Geometry check sheet. Reference: the model listing, model coordinates, mm. A direction names the side the tool comes from. Round coordinates to 2 decimals unless told otherwise and drop trailing zeros. Write each loop counter-clockwise with the first axis right and the second up, starting at its lowest first coordinate (ties: lowest second). Pieces come first, ordered by that corner, then holes. Notation, with made-up numbers: (20, 28.5) -> (37, 28.5) arc R14 cw to (37, 43.5) -> close; hole circle Ø3 at (4, 13). An arc over 180 degrees is marked (long way). Use a Markdown table: item, result.
```python
from build123d import *

# Parameters (mm, degrees)
BOSS_EXTRUDE1_DEPTH = 36
SKETCH2_R           = 1.6
CUT_EXTRUDE1_DEPTH  = 10
SKETCH3_R           = 1.95
CUT_EXTRUDE2_DEPTH  = 3
FILLET1_R           = 1
SKETCH4_W           = 8
SKETCH4_H           = 10.3
CUT_EXTRUDE3_DEPTH  = 10
SKETCH5_W           = 5.039372534
SKETCH5_H           = 10.3
CUT_EXTRUDE4_DEPTH  = 10


with BuildPart() as part:
    # Sketch1 → Boss-Extrude1 (new body)
    with BuildSketch(Plane.XY):
        Polygon((1.933806537, 5.15), (1.933806537, -5.15), (0.476512405, -5.15), (-2.040358106, -2.633129489), (-2.040358106, 2.633129489), (0.476512405, 5.15), align=None)
    extrude(amount=BOSS_EXTRUDE1_DEPTH)

    # Sketch2 → Cut-Extrude1 (cut)
    with BuildSketch(Plane(origin=(1.933806537, 0, 0), x_dir=(0, 0, -1), z_dir=(1, 0, 0))):
        with Locations((-16, 0)):
            Circle(SKETCH2_R)
        with Locations((-31, 0)):
            Circle(SKETCH2_R)
        with Locations((-6, 0)):
            Circle(SKETCH2_R)
    extrude(amount=-CUT_EXTRUDE1_DEPTH, mode=Mode.SUBTRACT)

    # Sketch3 → Cut-Extrude2 (cut)
    with BuildSketch(Plane.ZY.offset(2.040358106)):
        with Locations((16, 0)):
            Circle(SKETCH3_R)
        with Locations((31, 0)):
            Circle(SKETCH3_R)
        with Locations((6, 0)):
            Circle(SKETCH3_R)
    extrude(amount=-CUT_EXTRUDE2_DEPTH, mode=Mode.SUBTRACT)

    # Fillet1
    fillet1_edges = [part.edges().sort_by_distance(p)[0] for p in [
        (0.476512405, 5.15, 18),
        (0.476512405, -5.15, 18),
        (-2.040358106, 2.633129489, 18),
        (-2.040358106, -2.633129489, 18),
    ]]
    fillet(fillet1_edges, radius=FILLET1_R)

    # Sketch4 → Cut-Extrude3 (cut)
    with BuildSketch(Plane(origin=(1.933806537, 0, 0), x_dir=(0, 0, -1), z_dir=(1, 0, 0))):
        with Locations((-32, 0)):
            Rectangle(SKETCH4_W, SKETCH4_H)
    extrude(amount=-CUT_EXTRUDE3_DEPTH, mode=Mode.SUBTRACT)

    # Sketch5 → Cut-Extrude4 (cut)
    with BuildSketch(Plane(origin=(1.933806537, 0, 0), x_dir=(0, 0, -1), z_dir=(1, 0, 0))):
        with Locations((-25.480313733, 0)):
            Rectangle(SKETCH5_W, SKETCH5_H)
    extrude(amount=-CUT_EXTRUDE4_DEPTH, mode=Mode.SUBTRACT)


solid = part.part
```
(1) Section check D-D on z = 21. Record the cut outline in (x, y), plus the area to 3 significant figures.
A:
| item | result |
|---|---|
| outline | (-2.04, -2.22) arc R1 ccw to (-1.75, -2.93) -> (0.18, -4.86) arc R1 ccw to (0.89, -5.15) -> (1.93, -5.15) -> (1.93, 5.15) -> (0.89, 5.15) arc R1 ccw to (0.18, 4.86) -> (-1.75, 2.93) arc R1 ccw to (-2.04, 2.22) -> close |
| area | 34.5 mm2 |
(2) Section check A-A on z = 6. Record the cut outline in (x, y).
A:
| item | result |
|---|---|
| outline | (-2.04, -2.22) arc R1 ccw to (-1.75, -2.93) -> (0.18, -4.86) arc R1 ccw to (0.89, -5.15) -> (1.93, -5.15) -> (1.93, -1.6) -> (0.96, -1.6) -> (0.96, -1.95) -> (-2.04, -1.95) -> close; (-2.04, 1.95) -> (0.96, 1.95) -> (0.96, 1.6) -> (1.93, 1.6) -> (1.93, 5.15) -> (0.89, 5.15) arc R1 ccw to (0.18, 4.86) -> (-1.75, 2.93) arc R1 ccw to (-2.04, 2.22) -> close |
(3) Thickness scan on line 1 (Z direction, x = -0.1, y = 0.25); line 2 (Y direction, x = 1.4, z = 6); line 3 (Z direction, x = -0.25, y = -1.5). Record the ranges inside material, lowest first.
A:
| item | result |
|---|---|
| line 1 | z = 0 to 4.07, 7.93 to 14.07, 17.93 to 22.96 |
| line 2 | y = -5.15 to -1.6, 1.6 to 5.15 |
| line 3 | z = 0 to 4.75, 7.25 to 14.75, 17.25 to 22.96 |
(4) Gauge pin test, flat ends, axial feed: pin 1 Ø3 at (y, z) = (-3, 12) entering from -X; pin 2 Ø3 at (y, z) = (0, 6) entering from +X; pin 3 Ø1 at (x, z) = (-1, 18) entering from +Y. Record the tip position at first contact, or that the pin passes through.
A:
| item | result |
|---|---|
| pin 1 | stops at x = -2.04 |
| pin 2 | passes through |
| pin 3 | stops at y = 4.17 |
(5) Section check C-C on x = -0.5. Record the cut outline in (y, z).
A:
| item | result |
|---|---|
| outline | (-4.17, 0) -> (4.17, 0) -> (4.17, 22.96) -> (-4.17, 22.96) -> close; hole circle Ø3.9 at (0, 6); hole circle Ø3.9 at (0, 16) |
(6) Section check B-B on y = 0. Record the cut outline in (x, z).
A:
| item | result |
|---|---|
| outline | (-2.04, 0) -> (1.93, 0) -> (1.93, 4.4) -> (0.96, 4.4) -> (0.96, 4.05) -> (-2.04, 4.05) -> close; (-2.04, 7.95) -> (0.96, 7.95) -> (0.96, 7.6) -> (1.93, 7.6) -> (1.93, 14.4) -> (0.96, 14.4) -> (0.96, 14.05) -> (-2.04, 14.05) -> close; (-2.04, 17.95) -> (0.96, 17.95) -> (0.96, 17.6) -> (1.93, 17.6) -> (1.93, 22.96) -> (-2.04, 22.96) -> close |
(7) Access from +Z, -Z, +X, -X, +Y, -Y to the whole of each face (thin tool, end or side, straight path). Record for faces 1 (the face through (-0.795, 3.878, 11.32)), 2 (the face through (-0.561, 0.086, 14.052)).
A:
| item | result |
|---|---|
| face 1 | +Z, -Z, -X, +Y |
| face 2 | -X |
(8) Release check for a two-part mould opening along Y. For faces 3 (the face through (-0.561, 0.086, 4.052)), 4 (the face through (-0.768, -3.905, 11.32)), 5 (the face through (1.4, 5.15, 11.3)) record: +Y half, -Y half, draft (parallel to the pull), parting line (faces both ways), or undercut.
A:
| item | result |
|---|---|
| face 3 | undercut |
| face 4 | -Y half |
| face 5 | +Y half |
